Answer from the drawing. Dimensions are ordinates in mm from the lowest x, y and z of the part. A direction names the side the tool comes from. Round coordinates to 2 decimals unless told otherwise and drop trailing zeros. Loops run counter-clockwise (first coordinate to the right, second up) from the corner with the lowest first, then second, coordinate; pieces in that order, holes last. Notation, with made-up numbers: M 87.25,34.5 L 134.25,34.5 A19 cw 134.25,67.5 Z; hole C 83,-36.75 d5. An arc over 180 degrees is marked long. Answer as CSV lines item,"result".
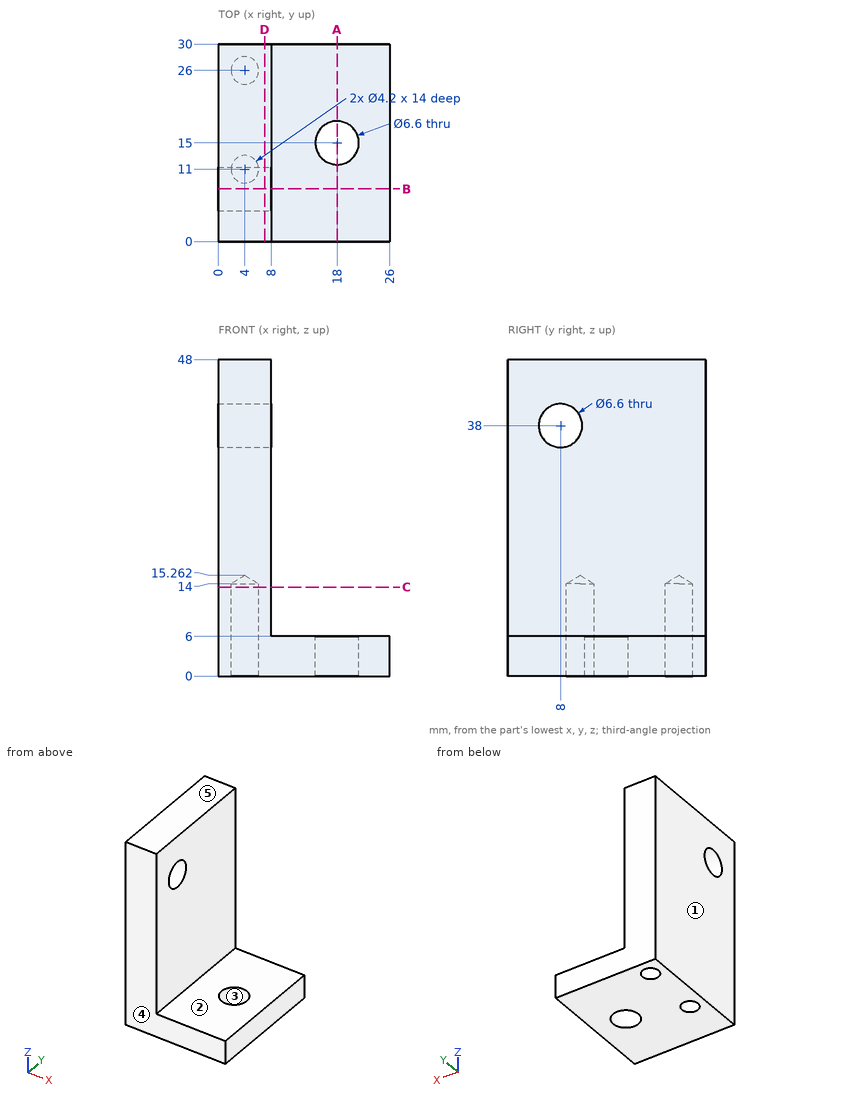
1) Each of these flat-tipped pins is pushed along its axis until it touches: P1, Ø14.5, axis at x = 16, y = 16, coming from the +Z side; P2, Ø9, axis at y = 17, z = 19, coming from the +X side. Where does it stop, or does it pass through?
Evaluation:
P1,"stops at z = 6"
P2,"stops at x = 8"
2) A tool of negligible diameter and unlimited length cuts with its end or side. For the marked faces 1 and 2, from which of +Z, -Z, +X, -X, +Y, -Y can it reach the whole face along a straight path? Write none if from no direction.
Evaluation:
face 1,"+Z, -Z, -X, +Y, -Y"
face 2,"+Z, +X, +Y, -Y"
3) Find section D-D, the plane x = 7. Give the vertices of the cut face in (y, z).
Evaluation:
outline,"M 0,0 L 30,0 L 30,48 L 0,48 Z; hole C 8,38 d6.6"
4) Straight lines are drawn through the part: line 1 (Y direction, x = 4, z = 10.25); line 2 (Y direction, x = 18, z = 3.5); line 3 (X direction, y = 15, z = 3.05). For each, find the intervals that lie inside material, in ascending order.
Evaluation:
line 1,"y = 0 to 8.9, 13.1 to 23.9, 28.1 to 30"
line 2,"y = 0 to 11.7, 18.3 to 30"
line 3,"x = 0 to 14.7, 21.3 to 26"
5) Find section B-B, the plane y = 8. Give the vertices of the cut face in (x, z), then the cut area to 3 significant figures.
Evaluation:
outline,"M 0,0 L 26,0 L 26,6 L 8,6 L 8,34.7 L 0,34.7 Z; M 0,41.3 L 8,41.3 L 8,48 L 0,48 Z"
area,"439 mm^2"
6) Determine the mould class of the marked faces 3, 4 and 5 for opening direction Y: released by +Y, released by -Y, zero draft, split by the parting line, or undercut.
Evaluation:
face 3,"undercut"
face 4,"released by -Y"
face 5,"zero draft"
7) Find section C-C, the plane z = 13.5. Give the vertices of the cut face in (x, y).
Evaluation:
outline,"M 0,0 L 8,0 L 8,30 L 0,30 Z; hole C 4,11 d4.2; hole C 4,26 d4.2"
8) Find section A-A, the plane x = 18. Give the vertices of the cut face in (y, z), then the cut area to 3 significant figures.
Evaluation:
outline,"M 0,0 L 11.7,0 L 11.7,6 L 0,6 Z; M 18.3,0 L 30,0 L 30,6 L 18.3,6 Z"
area,"140 mm^2"
